Autodesk Inventor part; units mm, degrees
ref_plane "YZ Plane" through (0, 0, 0) normal (1, 0, 0) x (0, 1, 0)
ref_plane "XZ Plane" through (0, 0, 0) normal (0, 1, 0) x (-1, 0, 0)
ref_plane "XY Plane" through (0, 0, 0) normal (0, 0, 1) x (1, 0, 0)
sketch "Szkic1" plane through (0, 0, 0) normal (0, 1, 0) x (-1, 0, 0)
  line L0 (0, 0) -> (0, -30)
  circle A0 centre (0, 0) radius 2
  circle A1 centre (0, -30) radius 2
  line L1 (0, 0) -> (0, -30) construction
  line L2 (-25, 0) -> (-25, -30)
  line L3 (25, -30) -> (25, 0)
  arc A2 (25, 0) -> (-25, 0) centre (0, 0) ccw
  arc A3 (-25, -30) -> (25, -30) centre (0, -30) ccw
  line L4 (-20.2, -40.2) -> (20.2, -40.2)
  line L5 (20.2, -40.2) -> (20.2, -19.8)
  line L6 (20.2, -19.8) -> (-20.2, -19.8)
  line L7 (-20.2, -19.8) -> (-20.2, -40.2)
  line L8 (-20.2, -40.2) -> (20.2, -19.8) construction
  line L9 (20.2, -40.2) -> (-20.2, -19.8) construction
  line L10 (0, -15) -> (-25, -15) construction
  line L11 (0, -30) -> (0, 0)
  circle A4 centre (0, 0) radius 2
  line L12 (0, -30) -> (0, 0) construction
  line L13 (-20.2, 10.2) -> (20.2, 10.2)
  line L14 (20.2, 10.2) -> (20.2, -10.2)
  line L15 (20.2, -10.2) -> (-20.2, -10.2)
  line L16 (-20.2, 10.2) -> (20.2, -10.2) construction
  line L17 (20.2, 10.2) -> (-20.2, -10.2) construction
  line L18 (-20.2, -10.2) -> (-20.2, 10.2)
  line L19 (0, -15) -> (-400, -15) construction
  line L20 (0, -15) -> (400, -15) construction
  dimension "d0" = 30
  dimension "d1" = 4
  dimension "d2" = 4
  dimension "d3" = 50
  dimension "d6" = 40.4
  dimension "d7" = 20.4
  dimension "d8" = 400
  dimension "d9" = 180
extrude "Wyciągnięcie proste1" add sketch "Szkic1" against normal blind 2 contours A2 L3 A3 L2
properties part number "base"
Geometry: final body of the model. Coordinates: model frame, mm. A direction names the side the tool comes from. Give positions to 0.01 mm unless a question says otherwise; leave off trailing zeros. Write each loop counter-clockwise with the first axis right and the second up, starting at its lowest first coordinate (ties: lowest second). Pieces come first, ordered by that corner, then holes.
(1) Access query for faces 1 (the flat face through (0, -2, -14)), 2 (the flat face through (0, -1, -10.2)). Directions: +Z, -Z, +X, -X, +Y, -Y. A direction counts if a zero-diameter tool reaches every point of the face in a straight line with its end or side. Return the directions, or none.
(2) Ray query, line 1 (Z direction, x = 0.5, y = -1.55) (3 decimals); line 2 (Z direction, x = -8.5, y = -1.05); line 3 (X direction, y = -0.35, z = -8). Return the intervals inside material, ascending.
(3) Cut plane B-B, the plane y = -0.4. Return loops of the section in (x, z).
(4) Cut plane C-C, the plane z = -27. Return loops of the section in (x, y).
(5) Cut plane A-A, the plane x = 7. Return loops of the section in (y, z).
(6) Cut plane D-D, the plane x = 0. Return loops of the section in (y, z), then the cut area to 3 significant figures.
(7) Mould query, pull axis Z, two halves, no side actions, for faces 3 (the flat face through (0, -1, -40.2)), 4 (the cylindrical face through (0.55, -0.986, -54.994)), 5 (the flat face through (25, -1, -15)), 6 (the flat face through (0, -1, 10.2)). Classes: released by +Z, released by -Z, zero draft, split by the parting line, or undercut.
(8) First-contact query: P1, Ø1, axis at x = 3.5, y = -1.5, coming from the +Z side; P2, Ø1, axis at x = 10, y = -1, coming from the -Z side; P3, Ø0.6, axis at y = -1.5, z = 3.5, coming from the -X side. Flat tips, straight axial feed; report the tip coordinate or a pass-through.
Values follow:
1. face 1: +Z, -Z, +X, -X, -Y
1. face 2: +Y, -Y
2. line 1: z = -54.995 to -40.2, -19.8 to -10.2, 10.2 to 24.995
2. line 2: z = -53.51 to -40.2, -19.8 to -10.2, 10.2 to 23.51
2. line 3: x = -25 to -20.2, 20.2 to 25
3. outline: (-25, -30) arc R25 ccw to (25, -30) - (25, 0) arc R25 ccw to (-25, 0) - close; hole (-20.2, -40.2) - (20.2, -40.2) - (20.2, -19.8) - (-20.2, -19.8) - close; hole (-20.2, -10.2) - (20.2, -10.2) - (20.2, 10.2) - (-20.2, 10.2) - close
4. outline: (-25, -2) - (-20.2, -2) - (-20.2, 0) - (-25, 0) - close; (20.2, -2) - (25, -2) - (25, 0) - (20.2, 0) - close
5. outline: (-2, -54) - (0, -54) - (0, -40.2) - (-2, -40.2) - close; (-2, -19.8) - (0, -19.8) - (0, -10.2) - (-2, -10.2) - close; (-2, 10.2) - (0, 10.2) - (0, 24) - (-2, 24) - close
6. outline: (-2, -55) - (0, -55) - (0, -40.2) - (-2, -40.2) - close; (-2, -19.8) - (0, -19.8) - (0, -10.2) - (-2, -10.2) - close; (-2, 10.2) - (0, 10.2) - (0, 25) - (-2, 25) - close
6. area: 78.4 mm2
7. face 3: undercut
7. face 4: released by -Z
7. face 5: zero draft
7. face 6: undercut
8. P1: stops at z = 24.82
8. P2: stops at z = -53.12
8. P3: stops at x = -24.79
